Work out the finished part from the listing and answer in its coordinate system (mm). A direction names the side the tool comes from. Give positions to 0.01 mm unless a question says otherwise; leave off trailing zeros. Loops run counter-clockwise (first coordinate to the right, second up) from the corner with the lowest first, then second, coordinate; pieces in that order, holes last. Notation, with made-up numbers: M 49,-12.75 L 54,-12.75 A20 cw 54,17.25 Z; hole C 77,41.5 d7. An arc over 180 degrees is marked long. Write item = value, one per line. Start each with the question number.
1. Section B-B on x = -16.5 is taken. Determine the outline of the cut face in (y, z).
2. Section A-A on z = 35 is taken. Determine the outline of the cut face in (x, y), plus the area to 3 significant figures.
3. The mould has two halves that part along Y. Classify faces 1 (the face through (23, -7, 22)), 2 (the face through (0, 0, 0)), 3 (the face through (7, 14, 3)): released by +Y, released by -Y, zero draft, split by the parting line, or undercut.
4. For faces 4 (the face through (-23, 7, 22)), 5 (the face through (-7, -14, 3)), 6 (the face through (0.1, 22.85, 22.74)), 7 (the face through (7, -23, 22)), 8 (the face through (-7, -23, 22)), determine the directions among +Z, -Z, +X, -X, +Y, -Y from which every point of the face is accessible in a straight line to the end or side of a thin tool.
5. Section D-D on x = 0 is taken. Determine the outline of the cut face in (y, z), plus the area to 4 significant figures.
6. Consider L1, parallel to Z at x = -21, y = 11.5; L2, parallel to X at y = 0.5, z = 26; L3, parallel to Y at x = -23, z = 33. Determine where each line is inside the solid, lowest interval first. Write a range as [from, to].
7. Flat-ended cylindrical pins translate along their axes: pin 1 Ø2.5 at (y, z) = (16.5, 3.5) entering from -X; pin 2 Ø12 at (x, z) = (-18, 18) entering from -Y; pin 3 Ø19.5 at (x, y) = (-19.5, 15.5) entering from +Z; pin 4 Ø1.5 at (y, z) = (-13, 1.5) entering from +X. Find the tip coordinate at first contact, or state that the pin passes through.
8. Section C-C on y = 13.5 is taken. Determine the outline of the cut face in (x, z).
Autodesk Fusion 360 part; units mm, degrees
sketch "スケッチ1" plane through (0, 0, 0) normal (0, 0, 1) x (1, 0, 0)
  circle A0 centre (0, 0) radius 25.5
  dimension "d1" = 51
extrude "押し出し1" add sketch "スケッチ1" along normal blind 40
sketch "スケッチ2" plane through (0, 0, 40) normal (0, 0, 1) x (-1, 0, 0)
  circle A0 centre (0, 0) radius 25.5
  circle A1 centre (0, 0) radius 22.85
  dimension "d4" = 45.7
extrude "押し出し2" cut sketch "スケッチ2" against normal blind 35 contours A1
sketch "スケッチ3" plane through (0, 0, 5) normal (0, 0, 1) x (-1, 0, 0)
  circle A0 centre (0, 0) radius 22.85
  line L0 (7, -7) -> (32, -7)
  line L1 (32, -7) -> (32, -32)
  line L2 (32, -32) -> (7, -32)
  line L3 (7, -32) -> (7, -7)
  line L4 (7, 7) -> (32, 7)
  line L5 (32, 7) -> (32, 32)
  line L6 (32, 32) -> (7, 32)
  line L7 (7, 32) -> (7, 7)
  line L8 (-7, 7) -> (-32, 7)
  line L9 (-32, 7) -> (-32, 32)
  line L10 (-32, 32) -> (-7, 32)
  line L11 (-7, 32) -> (-7, 7)
  line L12 (-7, -7) -> (-32, -7)
  line L13 (-32, -7) -> (-32, -32)
  line L14 (-32, -32) -> (-7, -32)
  line L15 (-7, -32) -> (-7, -7)
  dimension "d7" = 25
  dimension "d8" = 25
  dimension "d9" = 25
  dimension "d10" = 25
  dimension "d11" = 25
  dimension "d12" = 25
  dimension "d13" = 25
  dimension "d14" = 25
extrude "押し出し3" cut sketch "スケッチ3" along normal blind 35 contours A0 L12 L13 L14 L15
extrude "押し出し4" cut sketch "スケッチ3" along normal blind 35 contours A0 L0 L1 L2 L3
extrude "押し出し5" cut sketch "スケッチ3" along normal blind 35 contours A0 L4 L5 L6 L7 | A0 L8 L9 L10 L11
extrude "押し出し6" cut sketch "スケッチ3" against normal blind 5 contours A0 L4 L7 | A0 L0 L3 | A0 L8 L11 | A0 L12 L15
Verdict:
q1.outline = M -19.44,0 L -15.81,0 L -15.81,5 L -19.44,5 Z; M -7,0 L 7,0 L 7,5 L -7,5 Z; M 15.81,0 L 19.44,0 L 19.44,5 L 15.81,5 Z
q2.outline = M -24.52,-7 L -21.75,-7 A22.85 cw -21.75,7 L -24.52,7 A25.5 ccw Z; M -7,-24.52 A25.5 ccw 7,-24.52 L 7,-21.75 A22.85 cw -7,-21.75 Z; M -7,21.75 A22.85 cw 7,21.75 L 7,24.52 A25.5 ccw -7,24.52 Z; M 21.75,-7 L 24.52,-7 A25.5 ccw 24.52,7 L 21.75,7 A22.85 cw Z
q2.area = 151 mm2
q3.face_1 = released by -Y
q3.face_2 = zero draft
q3.face_3 = undercut
q4.face_4 = +Z, +X, -X, +Y
q4.face_5 = +Z, -Z
q4.face_6 = +Z
q4.face_7 = +Z, +X, +Y, -Y
q4.face_8 = +Z, -X, +Y, -Y
q5.outline = M -25.5,0 L 25.5,0 L 25.5,40 L 22.85,40 L 22.85,5 L -22.85,5 L -22.85,40 L -25.5,40 Z
q5.area = 440.5 mm2
q6.L1 = [0, 5]
q6.L2 = [-25.5, -22.84], [22.84, 25.5]
q6.L3 = [-7, 7]
q7.pin_1 = -20.44
q7.pin_2 = -7
q7.pin_3 = 40
q7.pin_4 = 22.36
q8.outline = M -21.63,0 L -18.44,0 L -18.44,5 L -21.63,5 Z; M -7,0 L 7,0 L 7,5 L -7,5 Z; M 18.44,0 L 21.63,0 L 21.63,5 L 18.44,5 Z
